Design review of the part shown in the three views and the two pictorial views. Dimensions are in mm from the part's minimum x, y and z. Coordinates: 2 decimals unless noted, no trailing zeros. Loops run counter-clockwise (first coordinate to the right, second up) from the corner with the lowest first, then second, coordinate; pieces in that order, holes last. Notation, with made-up numbers: (67.25, -25.5) -> (90.25, -25.5) arc R25 cw to (90.25, 10.5) -> close; hole circle Ø6 at (88.25, 55.5). An arc over 180 degrees is marked (long way). Use a Markdown table: item, result. Add a question column.
Q1. Draft analysis for pull direction X (two halves, no side actions). For the marked faces 1, 2 and 3, state which applies: pulls with the +X half, pulls with the -X half, needs draft (parallel to the pull), parting line crosses it, or undercut.
Q2. Take a section at D-D on z = 3.5. Write out the cut boundary in (x, y).
Q3. Clearance check with flat-ended pins moving along their axes: pin 1 Ø9.5 at (x, y) = (12, 6.5) entering from +Z; pin 2 Ø2 at (y, z) = (6, 2.5) entering from -X; pin 3 Ø3 at (y, z) = (12.5, 5.5) entering from +X; pin 4 Ø1 at (x, y) = (9, 8) entering from +Z. State where each tip first meets the part, or that it passes through.
Q4. For probe 1 along Y at (x, z) = (10, 2.05); probe 2 along Y at (x, z) = (10, 3.2); probe 3 along Z at (x, y) = (11.25, 16.25), list the stretches that pass through material, from the lowest coordinate up.
Q5. Take a section at A-A on y = 10. Write out the cut boundary in (x, z), plus the area to 3 significant figures.
Q6. Take a section at C-C on z = 1.25. Write out the cut boundary in (x, y).
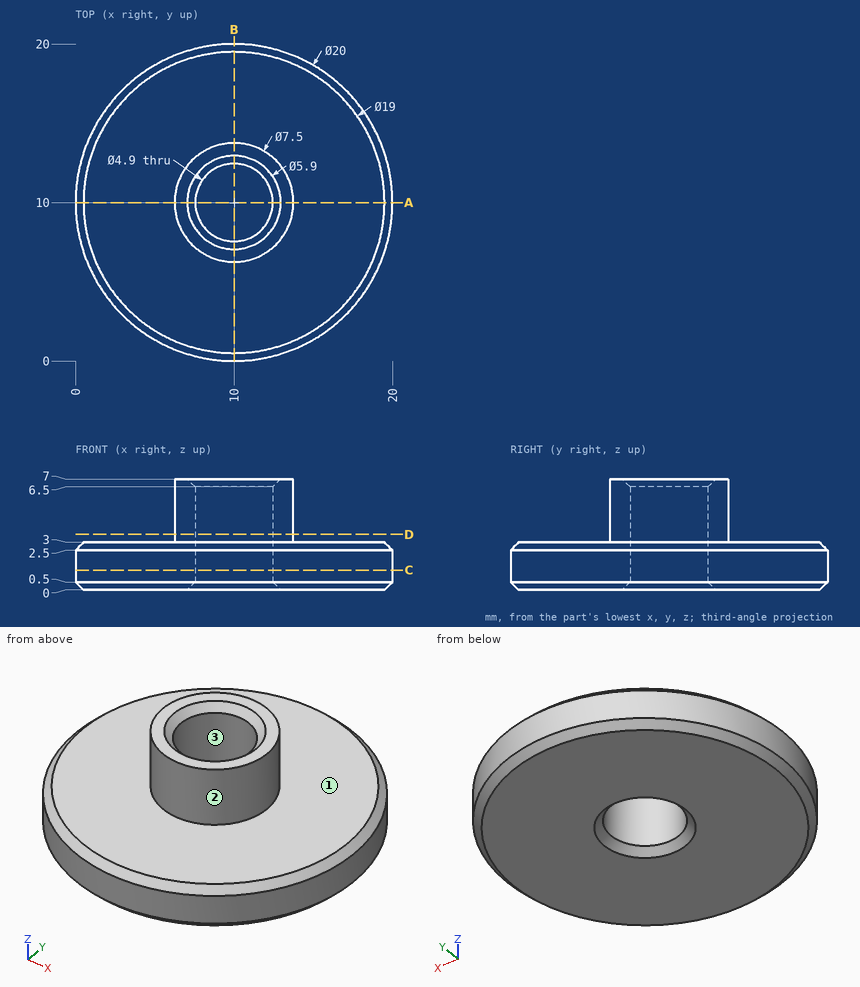
Answer list:
| question | item | result |
|---|---|---|
| 1 | face 1 | needs draft |
| 1 | face 2 | parting line crosses it |
| 1 | face 3 | undercut |
| 2 | outline | circle Ø7.5 at (10, 10); hole circle Ø4.9 at (10, 10) |
| 3 | pin 1 | z = 7 |
| 3 | pin 2 | x = 0.46 |
| 3 | pin 3 | x = 13.61 |
| 3 | pin 4 | z = 6.79 |
| 4 | probe 1 | 0 to 7.55, 12.45 to 20 |
| 4 | probe 2 | 6.25 to 7.55, 12.45 to 13.75 |
| 4 | probe 3 | 0 to 3 |
| 5 | outline | (0, 0.5) -> (0.5, 0) -> (7.05, 0) -> (7.55, 0.5) -> (7.55, 6.5) -> (7.05, 7) -> (6.25, 7) -> (6.25, 3) -> (0.5, 3) -> (0, 2.5) -> close; (12.45, 0.5) -> (12.95, 0) -> (19.5, 0) -> (20, 0.5) -> (20, 2.5) -> (19.5, 3) -> (13.75, 3) -> (13.75, 7) -> (12.95, 7) -> (12.45, 6.5) -> close |
| 5 | area | 54.7 mm² |
| 6 | outline | circle Ø20 at (10, 10); hole circle Ø4.9 at (10, 10) |
